Study the drawing (mm; zero at the part's minimum x, y, z) and answer. Round coordinates to 2 decimals unless told otherwise and drop trailing zeros. Order: outer loops, then holes, each group sorted by start corner. A loop starts at its lowest first (then second) coordinate and runs counter-clockwise, first axis right, second up. Notation, with made-up numbers: (24, 58.5) - (83, 58.5) arc R30 cw to (83, 91.5) - close; hole circle Ø7 at (19, 18). An arc over 180 degrees is marked (long way). Use one line per item in the form item = value. Start each with the question number.
Q1. The part is cut by section D-D on z = 22.5. Determine the outline of the cut face in (x, y).
Q2. Given P1, Ø2, axis at x = 172, z = 27.5, coming from the -Y side; P2, Ø4, axis at y = 186.5, z = 8.5, coming from the +X side; P3, Ø8, axis at x = 57, y = 100, coming from the -Z side; P4, Ø1.5, axis at y = 143.5, z = 36.5, coming from the -X side, each flat-ended and moving along its own axis, determine where each tip first touches the part or whether it passes through.
Q3. The part is cut by section C-C on x = 185. Determine the outline of the cut face in (y, z), plus the area to 3 significant figures.
Q4. Find the intervals of material crossed by line 1 (Y direction, x = 120, z = 20); line 2 (Y direction, x = 120, z = 29); line 3 (X direction, y = 186, z = 38), in increasing order. Write a range as [from, to].
Q5. The part is cut by section A-A on x = 120. Determine the outline of the cut face in (y, z), plus the area to 3 significant figures.
Q6. For a pull along Y with two mould halves and no side action, classify the marked faces 1 and 2 as +Y half, -Y half, draft (parallel to the pull), parting line (faces both ways), or undercut.
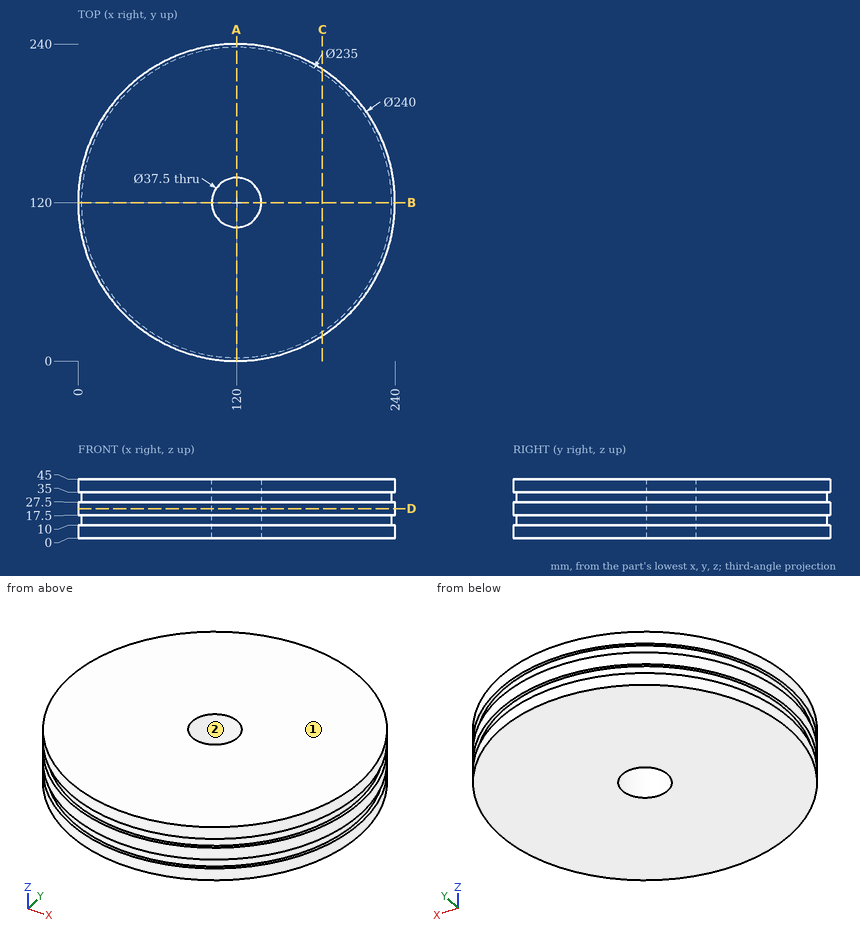
Found:
q1.outline = circle Ø240 at (120, 120); hole circle Ø37.5 at (120, 120)
q2.P1 = 11.38
q2.P2 = 221.19
q2.P3 = 0
q2.P4 = 2.18
q3.outline = (19.13, 0) - (220.87, 0) - (220.87, 10) - (217.88, 10) - (217.88, 17.5) - (220.87, 17.5) - (220.87, 27.5) - (217.88, 27.5) - (217.88, 35) - (220.87, 35) - (220.87, 45) - (19.13, 45) - (19.13, 35) - (22.12, 35) - (22.12, 27.5) - (19.13, 27.5) - (19.13, 17.5) - (22.12, 17.5) - (22.12, 10) - (19.13, 10) - close
q3.area = 8,990 mm²
q4.line_1 = [0, 101.25], [138.75, 240]
q4.line_2 = [2.5, 101.25], [138.75, 237.5]
q4.line_3 = [19.78, 220.22]
q5.outline = (0, 0) - (101.25, 0) - (101.25, 45) - (0, 45) - (0, 35) - (2.5, 35) - (2.5, 27.5) - (0, 27.5) - (0, 17.5) - (2.5, 17.5) - (2.5, 10) - (0, 10) - close; (138.75, 0) - (240, 0) - (240, 10) - (237.5, 10) - (237.5, 17.5) - (240, 17.5) - (240, 27.5) - (237.5, 27.5) - (237.5, 35) - (240, 35) - (240, 45) - (138.75, 45) - close
q5.area = 9,040 mm²
q6.face_1 = draft
q6.face_2 = undercut
